Input: part model. Units: mm. Frame: model coordinates. Round coordinates to 2 decimals unless told otherwise and drop trailing zeros. Loops run counter-clockwise (first coordinate to the right, second up) from the corner with the lowest first, then second, coordinate; pieces in that order, holes last. Notation, with made-up numbers: (31.5, -8.75) -> (86.5, -8.75) arc R32 ccw to (86.5, 30.25) -> close; hole circle Ø1 at (88.25, -34.75). An arc over 180 degrees is marked (long way). One line per question, with ' | ' between items. Start each with the question number.
Q1. Material intervals for L1, parallel to X at y = 0.6, z = -138; L2, parallel to X at y = 1.6, z = -55 (3 decimals); L3, parallel to X at y = 2.65, z = 12.5 (3 decimals), sorted ascending.
Q2. Contact query for flat-ended pins moving along their axis: P1, Ø1.6, axis at y = 2.5, z = -150.5, coming from the -X side; P2, Ø1, axis at y = 1, z = -150.5, coming from the +X side; P3, Ø1.6, axis at x = 619, y = 1, coming from the -Z side; P4, Ø4, axis at x = 22.93, z = 14.23, coming from the -Y side. Output: stop coordinate, or through.
Q3. Cut plane A-A on x = 303. Return loops of the section in (y, z) (3 decimals), and give its area (3 significant figures).
from build123d import *

# Parameters (mm, degrees)
SKETCH1_W           = 629.90984
SKETCH1_H           = 147.69846
BOSS_EXTRUDE1_DEPTH = 3.175
SKETCH3_W           = 254
SKETCH3_H           = 3.175
BOSS_EXTRUDE2_DEPTH = 6.35
SKETCH4_W           = 3.175
SKETCH4_H           = 188.732840052
CUT_EXTRUDE1_DEPTH  = 3.175
SKETCH9_W           = 3.175
SKETCH9_H           = 77.20584
BOSS_EXTRUDE4_DEPTH = 3.175
SKETCH10_W          = 636.25984
SKETCH10_H          = 24.39416
BOSS_EXTRUDE5_DEPTH = 3.175
SKETCH13_R          = 2.25
CUT_EXTRUDE3_DEPTH  = 652.56536379


with BuildPart() as part:
    # Sketch1 → Boss-Extrude1 (new body)
    with BuildSketch(Plane(origin=(0, 0, 0), x_dir=(1, 0, 0), z_dir=(0, 1, 0))):
        with Locations((314.95492, 73.84923)):
            Rectangle(SKETCH1_W, SKETCH1_H)
    extrude(amount=BOSS_EXTRUDE1_DEPTH)

    # Sketch3 → Boss-Extrude2 (add)
    with BuildSketch(Plane(origin=(0, 0, -147.69846), x_dir=(-1, 0, 0), z_dir=(0, 0, -1))):
        with Locations((-473.22613, 1.5875)):
            Rectangle(SKETCH3_W, SKETCH3_H)
        with Locations((-156.68371, 1.5875)):
            Rectangle(SKETCH3_W, SKETCH3_H)
    extrude(amount=BOSS_EXTRUDE2_DEPTH)

    # Sketch4 → Cut-Extrude1 (cut)
    with BuildSketch(Plane(origin=(0, 3.175, 0), x_dir=(1, 0, 0), z_dir=(0, 1, 0))):
        with Locations((314.95492, 147.69846)):
            Rectangle(SKETCH4_W, SKETCH4_H)
    extrude(amount=-CUT_EXTRUDE1_DEPTH, mode=Mode.SUBTRACT)

    # Sketch9 → Boss-Extrude4 (add, through all)
    with BuildSketch(Plane.XZ):
        with Locations((-1.5875, -38.60292)):
            Rectangle(SKETCH9_W, SKETCH9_H)
        with Locations((631.49734, -38.60292)):
            Rectangle(SKETCH9_W, SKETCH9_H)
    extrude(amount=-BOSS_EXTRUDE4_DEPTH)

    # Sketch10 → Boss-Extrude5 (add, through all)
    with BuildSketch(Plane(origin=(0, 3.175, 0), x_dir=(1, 0, 0), z_dir=(0, 1, 0))):
        with Locations((314.95492, -12.19708)):
            Rectangle(SKETCH10_W, SKETCH10_H)
    extrude(amount=-BOSS_EXTRUDE5_DEPTH)

    # Sketch13 → Cut-Extrude3 (cut, through all)
    with BuildSketch(Plane(origin=(0, 3.175, 0), x_dir=(1, 0, 0), z_dir=(0, 1, 0))):
        with Locations(Location((606.977733219, -14.23416, 0), (0, 0, 270))):
            Circle(SKETCH13_R)
        with Locations(Location((460.966326609, -14.23416, 0), (0, 0, 270))):
            Circle(SKETCH13_R)
        with Locations(Location((314.95492, -14.23416, 0), (0, 0, 270))):
            Circle(SKETCH13_R)
        with Locations(Location((168.943513391, -14.23416, 0), (0, 0, 270))):
            Circle(SKETCH13_R)
        with Locations(Location((22.932106781, -14.23416, 0), (0, 0, 270))):
            Circle(SKETCH13_R)
    extrude(amount=-CUT_EXTRUDE3_DEPTH, mode=Mode.SUBTRACT)


solid = part.part
Results:
1) L1: 0 to 313.37, 316.54 to 629.91 | L2: -3.175 to 313.367, 316.542 to 633.085 | L3: -3.175 to 21.499, 24.366 to 167.51, 170.377 to 313.521, 316.389 to 459.533, 462.4 to 605.544, 608.411 to 633.085
2) P1: x = 29.68 | P2: x = 600.23 | P3: z = -147.7 | P4: through
3) outline: (0, -147.698) -> (3.175, -147.698) -> (3.175, 24.394) -> (0, 24.394) -> close | area: 546 mm^2
